Model file for the job. Use its own axes, mm. Face numbers are marked on the shaded views. Coordinates: 2 decimals unless noted, no trailing zeros. Write each loop counter-clockwise with the first axis right and the second up, starting at its lowest first coordinate (ties: lowest second). Pieces come first, ordered by that corner, then holes.
Q1. Band-saw the part on A-A, the plane y = 0. Write the cut outline in (x, z).
Q2. Drill centre lines: probe 1 along X at (y, z) = (0, 0.15); probe 2 along X at (y, z) = (-3.75, 0.5); probe 3 along Y at (x, z) = (0, -0.3). Where is each one in solid material? Low to high.
Q3. Pull direction Y, two halves, no side cores. Call the marked faces 1 and 2: released by +Y, released by -Y, zero draft, split by the parting line, or undercut.
Q4. Band-saw the part on D-D, the plane y = 4.5. Write the cut outline in (x, z), plus the area to 4 significant figures.
Q5. Band-saw the part on B-B, the plane x = 0. Write the cut outline in (y, z), plus the area to 4 significant figures.
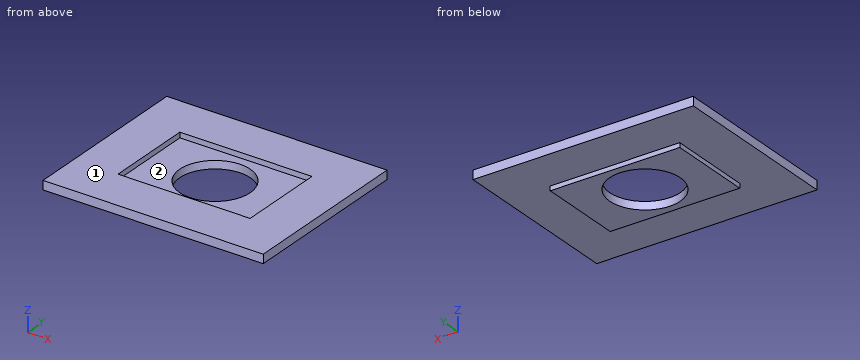
from build123d import *

# Parameters (mm, degrees)
F0_W     = 25
F0_H     = 20
F0_R     = 4
F1_DEPTH = 1
F2_W     = 15
F2_H     = 10
F3_DEPTH = 0.6
F4_W     = 14.7
F4_H     = 9.7
F4_R     = 4
F5_DEPTH = 0.5


with BuildPart() as f1:
    # F0 (on Top) → F1 (new body)
    with BuildSketch(Plane.XY):
        Rectangle(F0_W, F0_H)
        Circle(F0_R, mode=Mode.SUBTRACT)
    extrude(amount=F1_DEPTH)

    # F2 (on face) → F3 (cut)
    with BuildSketch(Plane.XY.offset(1)):
        Rectangle(F2_W, F2_H)
    extrude(amount=-F3_DEPTH, mode=Mode.SUBTRACT)

    # F4 (on face) → F5 (join)
    with BuildSketch(Plane(origin=(0, 0, 0), x_dir=(1, 0, 0), z_dir=(0, 0, -1))):
        Rectangle(F4_W, F4_H)
        Circle(F4_R, mode=Mode.SUBTRACT)
    extrude(amount=F5_DEPTH)


solid = f1.part
Answer sheet:
1. outline: (-12.5, 0) - (-7.35, 0) - (-7.35, -0.5) - (-4, -0.5) - (-4, 0.4) - (-7.5, 0.4) - (-7.5, 1) - (-12.5, 1) - close; (4, -0.5) - (7.35, -0.5) - (7.35, 0) - (12.5, 0) - (12.5, 1) - (7.5, 1) - (7.5, 0.4) - (4, 0.4) - close
2. probe 1: x = -12.5 to -4, 4 to 12.5
2. probe 2: x = -12.5 to -7.5, 7.5 to 12.5
2. probe 3: y = -4.85 to -4, 4 to 4.85
3. face 1: zero draft
3. face 2: undercut
4. outline: (-12.5, 0) - (-7.35, 0) - (-7.35, -0.5) - (7.35, -0.5) - (7.35, 0) - (12.5, 0) - (12.5, 1) - (7.5, 1) - (7.5, 0.4) - (-7.5, 0.4) - (-7.5, 1) - (-12.5, 1) - close
4. area: 23.35 mm2
5. outline: (-10, 0) - (-4.85, 0) - (-4.85, -0.5) - (-4, -0.5) - (-4, 0.4) - (-5, 0.4) - (-5, 1) - (-10, 1) - close; (4, -0.5) - (4.85, -0.5) - (4.85, 0) - (10, 0) - (10, 1) - (5, 1) - (5, 0.4) - (4, 0.4) - close
5. area: 11.65 mm2
